Here's how the part is built. I have some questions about the finished solid (model axes, mm). A direction names the side the tool comes from. Round coordinates to 2 decimals unless told otherwise and drop trailing zeros. Order: outer loops, then holes, each group sorted by start corner. A loop starts at its lowest first (then second) coordinate and runs counter-clockwise, first axis right, second up.
Autodesk Fusion 360 part; units mm, degrees
sketch "Sketch1" plane through (0, 0, 0) normal (0, 0, 1) x (1, 0, 0)
  line L0 (0, 25) -> (25, 25)
  line L1 (25, 25) -> (25, 7.5)
  arc A0 (25, 7.5) -> (27.5, 5) centre (27.5, 7.5) ccw
  line L2 (27.5, 5) -> (100, 5)
  line L3 (100, 5) -> (100, 0)
  line L4 (0, 0) -> (0, 25) construction
  line L5 (0, 0) -> (100, 0) construction
  line L6 (0, -25) -> (25, -25)
  line L7 (25, -25) -> (25, -7.5)
  arc A1 (27.5, -5) -> (25, -7.5) centre (27.5, -7.5) ccw
  line L8 (27.5, -5) -> (100, -5)
  line L9 (100, -5) -> (100, 0)
  line L10 (0, 25) -> (-25, 25)
  line L11 (-25, 25) -> (-25, 7.5)
  arc A2 (-27.5, 5) -> (-25, 7.5) centre (-27.5, 7.5) ccw
  line L12 (-27.5, 5) -> (-100, 5)
  line L13 (-25, -25) -> (-25, -7.5)
  line L14 (-27.5, -5) -> (-100, -5)
  arc A3 (-25, -7.5) -> (-27.5, -5) centre (-27.5, -7.5) ccw
  line L15 (0, -25) -> (-25, -25)
  line L16 (-100, 5) -> (-100, 0)
  line L17 (-100, -5) -> (-100, 0)
  dimension "Fillet_Radius" = 2.5
  dimension "Shoulder_Height" = 20
  dimension "Shoulder_Width" = 50
  dimension "Total_Width" = 200
  dimension "Total_Height" = 50
extrude "Extrude1" add sketch "Sketch1" along normal mid plane 10
1. I'm going to push flat-ended pins straight in: P1, Ø5, axis at y = -17.5, z = 1.5, coming from the +X side; P2, Ø3, axis at x = 56.5, z = -0.5, coming from the +Y side; P3, Ø3, axis at x = -78, z = 2, coming from the -Y side. Where does each tip first touch, or does it pass through?
Evaluation:
P1: stops at x = 25
P2: stops at y = 5
P3: stops at y = -5
2. On a 3-axis mill with a long thin cutter (end or side, diameter ignored), from which of +Z, -Z, +X, -X, +Y, -Y can I reach the whole of each face in a straight line? I mean faces 1 (the flat face through (63, 5, 0)), 2 (the flat face through (-25, -16, 0)), 3 (the flat face through (-63, 5, 0)), 4 (the flat face through (63, -5, 0)). Say none if no direction works.
Evaluation:
face 1: +Z, -Z, +X, +Y
face 2: +Z, -Z, -X, -Y
face 3: +Z, -Z, -X, +Y
face 4: +Z, -Z, +X, -Y
3. I need wall thicknesses on probe 1 along X at (y, z) = (-10.5, 0.25); probe 2 along Y at (x, z) = (-30, -3.5); probe 3 along X at (y, z) = (6, 0.75). Which ranges of each line are inside material? Lowest first, please.
Evaluation:
probe 1: x = -25 to 25
probe 2: y = -5 to 5
probe 3: x = -25.5 to 25.5
4. If we section it at C-C, the plane y = 12: Write out the boundary of the cut face in (x, z).
Evaluation:
outline: (-25, -5) - (25, -5) - (25, 5) - (-25, 5) - close
5. If we section it at A-A, the plane z = -3.5: Write out the boundary of the cut face in (x, y), and give its area (3 significant figures).
Evaluation:
outline: (-100, -5) - (-27.5, -5) arc R2.5 cw to (-25, -7.5) - (-25, -25) - (25, -25) - (25, -7.5) arc R2.5 cw to (27.5, -5) - (100, -5) - (100, 5) - (27.5, 5) arc R2.5 cw to (25, 7.5) - (25, 25) - (-25, 25) - (-25, 7.5) arc R2.5 cw to (-27.5, 5) - (-100, 5) - close
area: 4,010 mm2
6. If we section it at B-B, the plane x = -72: Write out the boundary of the cut face in (y, z), and give its area (3 significant figures).
Evaluation:
outline: (-5, -5) - (5, -5) - (5, 5) - (-5, 5) - close
area: 100 mm2
